Could you check a few things on this model? Use its own coordinates, in mm. Give positions to 0.01 mm unless a question says otherwise; leave off trailing zeros. Write each loop counter-clockwise with the first axis right and the second up, starting at its lowest first coordinate (ties: lowest second). Pieces come first, ordered by that corner, then holes. Notation, with made-up numbers: (-38.5, 56) - (6.5, 56) arc R25 ccw to (6.5, 79) - close; hole circle Ø5 at (31, -14.5). An arc over 180 degrees is marked (long way). Answer as a JSON object with one key per item and string values. Group by question number.
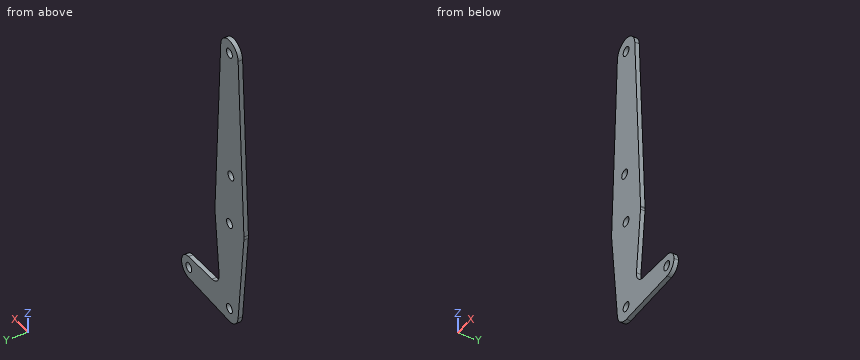
```python
from build123d import *

# Parameters (mm, degrees)
F0_R     = 3.175
F1_DEPTH = 3.048


with BuildPart() as f1:
    # F0 (on Front) → F1 (new body)
    with BuildSketch(Plane.XZ):
        with BuildLine():
            ThreePointArc((0.340179, -9.518923), (6.854408, -6.613827), (9.525, 0))
            ThreePointArc((9.525, 0), (-0.476848, 9.513056), (-9.477255, -0.9525))
            ThreePointArc((-9.477255, -0.9525), (-6.262383, -7.17692), (0.340179, -9.518923))
        make_face()
        Circle(F0_R, mode=Mode.SUBTRACT)
        with BuildLine():
            ThreePointArc((-9.477255, -0.9525), (-0.476848, 9.513056), (9.525, 0))
            ThreePointArc((9.525, 0), (6.854408, -6.613827), (0.340179, -9.518923))
            Line((0.340179, -9.518923), (44.733482, -7.932436))
            ThreePointArc((44.733482, -7.932436), (36.5125, 0), (44.733482, 7.932436))
            Line((44.733482, 7.932436), (18.9676, 8.853234))
            ThreePointArc((18.9676, 8.853234), (13.2612, 11.571359), (11.341187, 17.593382))
            Line((11.341187, 17.593382), (15.795426, 61.9125))
            ThreePointArc((15.795426, 61.9125), (0, 47.625), (-15.795426, 61.9125))
            Line((-15.795426, 61.9125), (-9.477255, -0.9525))
        make_face()
        with BuildLine():
            ThreePointArc((-15.855144, 64.29375), (-15.87001, 63.102003), (-15.795426, 61.9125))
            ThreePointArc((-15.795426, 61.9125), (0, 47.625), (15.795426, 61.9125))
            ThreePointArc((15.795426, 61.9125), (15.855094, 62.705253), (15.875, 63.5))
            ThreePointArc((15.875, 63.5), (15.870035, 63.896999), (15.855144, 64.29375))
            ThreePointArc((15.855144, 64.29375), (0, 79.375), (-15.855144, 64.29375))
        make_face()
        with Locations((0, 63.5)):
            Circle(F0_R, mode=Mode.SUBTRACT)
        with BuildLine():
            ThreePointArc((44.733482, 7.932436), (36.5125, 0), (44.733482, -7.932436))
            ThreePointArc((44.733482, -7.932436), (50.162007, -5.511523), (52.3875, 0))
            ThreePointArc((52.3875, 0), (50.162007, 5.511523), (44.733482, 7.932436))
        make_face()
        with Locations((44.45, 0)):
            Circle(F0_R, mode=Mode.SUBTRACT)
        with BuildLine():
            Line((-9.513086, 190.97625), (-15.855144, 64.29375))
            ThreePointArc((-15.855144, 64.29375), (0, 79.375), (15.855144, 64.29375))
            Line((15.855144, 64.29375), (9.513086, 190.97625))
            ThreePointArc((9.513086, 190.97625), (9.522021, 190.738199), (9.525, 190.5))
            ThreePointArc((9.525, 190.5), (-0.238199, 180.977979), (-9.513086, 190.97625))
        make_face()
        with Locations((-1.5875, 100.0252)):
            Circle(F0_R, mode=Mode.SUBTRACT)
        with BuildLine():
            ThreePointArc((9.513086, 190.97625), (0, 200.025), (-9.513086, 190.97625))
            ThreePointArc((-9.513086, 190.97625), (-0.238199, 180.977979), (9.525, 190.5))
            ThreePointArc((9.525, 190.5), (9.522021, 190.738199), (9.513086, 190.97625))
        make_face()
        with Locations((0, 190.5)):
            Circle(F0_R, mode=Mode.SUBTRACT)
    extrude(amount=F1_DEPTH)


solid = f1.part
```
(1) I need wall thicknesses on L1, parallel to Z at x = 44.45, y = -0.9 (3 decimals); L2, parallel to Z at x = -2.5, y = -1.35; L3, parallel to Z at x = 42.5, y = -2.9. Which ranges of each line are inside material? Lowest first, please.
(2) I want a section at B-B, the plane z = 108. Please give me the cut outline in (x, y), and give its area (3 significant figures).
(3) I want a section at C-C, the plane x = 7. Please give me the cut outline in (y, z), and give its area (3 significant figures).
(4) Will this pin go through, and if not, where does the flat tip stop? P1, Ø5.5, axis at x = 0, z = 0, coming from the +Y side.
(5) I want a section at A-A, the plane y = -1.8. State how many separate pieces and enclosed holes the cut face has, and give its area (3 significant figures).
Entries:
{
 "1": {"L1": "-7.943 to -3.175, 3.175 to 7.943", "L2": "-9.19 to -1.96, 1.96 to 61.54, 65.46 to 96.98, 103.07 to 188.54, 192.46 to 199.69", "L3": "-8.01 to -2.51, 2.51 to 8.01"},
 "2": {"outline": "(-13.67, -3.05) - (13.67, -3.05) - (13.67, 0) - (-13.67, 0) - close", "area": "83.3 mm^2"},
 "3": {"outline": "(-3.05, -9.28) - (0, -9.28) - (0, 196.96) - (-3.05, 196.96) - close", "area": "629 mm^2"},
 "4": {"P1": "through"},
 "5": {"separate pieces": "1", "enclosed holes": "5", "area": "5,700 mm^2"}
}
